from build123d import *

# Parameters (mm, degrees)
F0_R     = 6.35
F1_DEPTH = 6.35
F2_R     = 25.4
F3_R     = 5.08
F4_DEPTH = 19.05


with BuildPart() as f1:
    # F0 (on Front) → F1 (new body)
    with BuildSketch(Plane.XZ):
        with BuildLine():
            Line((-44.45, -31.75), (44.45, -31.75))
            Line((44.45, -31.75), (44.45, 31.75))
            Line((44.45, 31.75), (12.022284, 31.75))
            ThreePointArc((12.022284, 31.75), (10.258949, 23.22823), (6.357251, 15.449627))
            ThreePointArc((6.357251, 15.449627), (-3.659439, 12.571452), (-5.888707, 22.752234))
            ThreePointArc((-5.888707, 22.752234), (-3.139666, 26.882916), (-2.174649, 31.75))
            Line((-2.174649, 31.75), (-44.45, 31.75))
            Line((-44.45, 31.75), (-44.45, -31.75))
        make_face()
        with Locations((26.500253, -8.66654)):
            Circle(F0_R, mode=Mode.SUBTRACT)
        with Locations((26.500253, -8.66654)):
            Circle(F0_R)
    extrude(amount=F1_DEPTH)

    # F2
    f2_edges = [f1.edges().sort_by_distance(p)[0] for p in [
        (44.45, -3.175, -31.75),
        (44.45, -3.175, 31.75),
    ]]
    fillet(f2_edges, radius=F2_R)

    # F3
    f3_edges = [f1.edges().sort_by_distance(p)[0] for p in [
        (-44.45, -3.175, 31.75),
        (-44.45, -3.175, -31.75),
    ]]
    fillet(f3_edges, radius=F3_R)

    # F0 (on Front) → F4 (join)
    with BuildSketch(Plane.XZ):
        with Locations((26.500253, -8.66654)):
            Circle(F0_R)
    extrude(amount=F4_DEPTH)


solid = f1.part
Geometry check sheet. Reference: the model listing, model coordinates, mm. A direction names the side the tool comes from. Give positions to 0.01 mm unless a question says otherwise; leave off trailing zeros. Write each loop counter-clockwise with the first axis right and the second up, starting at its lowest first coordinate (ties: lowest second). Pieces come first, ordered by that corner, then holes. Notation, with made-up numbers: (47, 70) - (53, 70) arc R20 cw to (53, 74) - close; hole circle Ø1 at (51, 18). An arc over 180 degrees is marked (long way). Put each result on its own line as item: value.
1. Go/stop test with flat-tipped pins: pin 1 (4 mm diameter, centred on x = 33, y = -14, fed in from -Z); pin 2 (8 mm diameter, centred on x = -30.5, z = 15.5, fed in from -Y); pin 3 (8 mm diameter, centred on x = 32.5, y = -12, fed in from +Z); pin 4 (1 mm diameter, centred on y = -7, z = -18, fed in from +X). Record where each tip stops, or that it passes through.
Ans:
pin 1: stops at z = -13.15
pin 2: stops at y = -6.35
pin 3: stops at z = -2.64
pin 4: passes through
2. Sectioned sample at D-D, the plane z = 1. Enter the section's corners in (x, y).
Ans:
outline: (-44.45, -6.35) - (44.45, -6.35) - (44.45, 0) - (-44.45, 0) - close
3. Sectioned sample at A-A, the plane y = -3.75. Enter the section's corners in (x, z).
Ans:
outline: (-44.45, -26.67) arc R5.08 ccw to (-39.37, -31.75) - (19.05, -31.75) arc R25.4 ccw to (44.45, -6.35) - (44.45, 6.35) arc R25.4 ccw to (19.05, 31.75) - (12.02, 31.75) arc R33.45 cw to (6.36, 15.45) arc R7.14 cw (long way) to (-5.89, 22.75) arc R12.76 ccw to (-2.17, 31.75) - (-39.37, 31.75) arc R5.08 ccw to (-44.45, 26.67) - close
4. Draft check along X on faces 1 (the cylindrical face through (-42.922, -3.219, -30.301)), 2 (the flat face through (-1, 0, 0)), 3 (the cylindrical face through (-3.167, -3.131, 26.818)). Enter one of: +X half, -X half, draft (parallel to the pull), parting line (faces both ways), or undercut.
Ans:
face 1: -X half
face 2: draft
face 3: undercut
5. Sectioned sample at B-B, the plane z = 18. Enter the section's corners in (x, y), plus the area to 3 significant figures.
Ans:
outline: (-44.45, -6.35) - (-7.11, -6.35) - (-7.11, 0) - (-44.45, 0) - close; (7.92, -6.35) - (41.62, -6.35) - (41.62, 0) - (7.92, 0) - close
area: 451 mm²
6. Thickness scan on line 1 (Y direction, x = 33, z = -4); line 2 (Z direction, x = 19.5, y = -4.5); line 3 (Z direction, x = 2.5, y = -5.75). Record the ranges inside material, lowest first.
Ans:
line 1: y = -6.35 to 0
line 2: z = -31.75 to 31.75
line 3: z = -31.75 to 12.02
7. Set-up check for faces 4 (the cylindrical face through (-3.52, -3.13, 12.49)), 5 (the cylindrical face through (10.299, -3.131, 23.344)), 6 (the cylindrical face through (32.557, -12.611, -6.759)): record each of +Z, -Z, +X, -X, +Y, -Y from which the full face is reachable in a straight line by a thin tool's end or side.
Ans:
face 4: +Y, -Y
face 5: +Z, +Y, -Y
face 6: -Y
8. Sectioned sample at C-C, the plane x = 24. Enter the section's corners in (y, z), plus the area to 3 significant figures.
Ans:
outline: (-19.05, -14.5) - (-6.35, -14.5) - (-6.35, -31.26) - (0, -31.26) - (0, 31.26) - (-6.35, 31.26) - (-6.35, -2.83) - (-19.05, -2.83) - close
area: 545 mm²
